from build123d import *

# Parameters (mm, degrees)
SKETCH1_R           = 1.725
SKETCH1_R_2         = 3
BOSS_EXTRUDE3_DEPTH = 6
CUT_EXTRUDE1_DEPTH  = 4
FILLET1_R           = 4


with BuildPart() as part:
    # Sketch1 → Boss-Extrude3 (new body)
    with BuildSketch(Plane.XY):
        with BuildLine():
            ThreePointArc((22.418161887, -16.775756842), (28, 0), (22.418161887, 16.775756842))
            ThreePointArc((22.418161887, 16.775756842), (22.627416998, 22.627416998), (16.775756842, 22.418161887))
            ThreePointArc((16.775756842, 22.418161887), (0, 28), (-16.775756842, 22.418161887))
            ThreePointArc((-16.775756842, 22.418161887), (-22.627416998, 22.627416998), (-22.418161887, 16.775756842))
            ThreePointArc((-22.418161887, 16.775756842), (-28, 0), (-22.418161887, -16.775756842))
            ThreePointArc((-22.418161887, -16.775756842), (-22.627416998, -22.627416998), (-16.775756842, -22.418161887))
            ThreePointArc((-16.775756842, -22.418161887), (0, -28), (16.775756842, -22.418161887))
            ThreePointArc((16.775756842, -22.418161887), (22.627416998, -22.627416998), (22.418161887, -16.775756842))
        make_face()
        with Locations((-19.798989873, 19.798989873)):
            Circle(SKETCH1_R, mode=Mode.SUBTRACT)
        with Locations((19.798989873, 19.798989873)):
            Circle(SKETCH1_R, mode=Mode.SUBTRACT)
        with Locations((-19.798989873, -19.798989873)):
            Circle(SKETCH1_R, mode=Mode.SUBTRACT)
        with Locations((19.798989873, -19.798989873)):
            Circle(SKETCH1_R, mode=Mode.SUBTRACT)
        Circle(SKETCH1_R_2, mode=Mode.SUBTRACT)
        with Locations((0, 7.5)):
            Circle(SKETCH1_R, mode=Mode.SUBTRACT)
        with Locations((-7.5, 0)):
            Circle(SKETCH1_R, mode=Mode.SUBTRACT)
        with Locations((0, -7.5)):
            Circle(SKETCH1_R, mode=Mode.SUBTRACT)
        with Locations((7.5, 0)):
            Circle(SKETCH1_R, mode=Mode.SUBTRACT)
    extrude(amount=BOSS_EXTRUDE3_DEPTH)

    # Sketch2 → Cut-Extrude1 (cut)
    with BuildSketch(Plane.XY.offset(6)):
        Polygon((3.290896534, 7.5), (1.645448267, 10.35), (-1.645448267, 10.35), (-3.290896534, 7.5), (-1.645448267, 4.65), (1.645448267, 4.65), align=None)
        Polygon((-4.65, 1.645448267), (-7.5, 3.290896534), (-10.35, 1.645448267), (-10.35, -1.645448267), (-7.5, -3.290896534), (-4.65, -1.645448267), align=None)
        Polygon((10.35, -1.645448267), (10.35, 1.645448267), (7.5, 3.290896534), (4.65, 1.645448267), (4.65, -1.645448267), (7.5, -3.290896534), align=None)
        Polygon((3.290896534, -7.5), (1.645448267, -4.65), (-1.645448267, -4.65), (-3.290896534, -7.5), (-1.645448267, -10.35), (1.645448267, -10.35), align=None)
    extrude(amount=-CUT_EXTRUDE1_DEPTH, mode=Mode.SUBTRACT)

    # Fillet1
    fillet1_edges = [part.edges().sort_by_distance(p)[0] for p in [
        (22.418161887, 16.775756842, 3),
        (22.418161887, -16.775756842, 3),
        (16.775756842, -22.418161887, 3),
        (-16.775756842, -22.418161887, 3),
        (-22.418161887, -16.775756842, 3),
        (-22.418161887, 16.775756842, 3),
        (-16.775756842, 22.418161887, 3),
        (16.775756842, 22.418161887, 3),
    ]]
    fillet(fillet1_edges, radius=FILLET1_R)


solid = part.part
Can you work these out from the model? Positions are in its coordinate system, mm. A direction names the side the tool comes from. Coordinates: 2 decimals unless noted, no trailing zeros. Write each loop counter-clockwise with the first axis right and the second up, starting at its lowest first coordinate (ties: lowest second). Pieces come first, ordered by that corner, then holes. Notation, with made-up numbers: (38.5, 78.5) -> (49.5, 78.5) arc R31 ccw to (49.5, 102.5) -> close; hole circle Ø6 at (-22.5, -8). An arc over 180 degrees is marked (long way). Write each question's results on one line, items separated by ' | '. Start each with the question number.
Item 1: Thinking about a two-plate mould opening in Y: for faces 3 (the flat face through (6, -6, 0)), 4 (the flat face through (-8.94, -2.46, 4.03)), 5 (the cylindrical face through (0, 28, 3)), 6 (the flat face through (-6.06, 2.46, 4.03)), which applies, released by +Y, released by -Y, zero draft, split by the parting line, or undercut?
Item 2: If we section it at B-B, the plane x = 6.5: Write out the boundary of the cut face in (y, z), and give its area (3 significant figures).
Item 3: If we section it at C-C, the plane y = 1: Write out the boundary of the cut face in (x, z), and give its area (3 significant figures).
Item 4: Please list where these lines run through material, in increasing order: probe 1 along Y at (x, z) = (0, 0.8) (3 decimals); probe 2 along Y at (x, z) = (0, 2.6); probe 3 along X at (y, z) = (1, 5.5).
Item 5: If we section it at A-A, the plane x = 0: Write out the boundary of the cut face in (y, z) (3 decimals).
Item 6: I'm going to push flat-ended pins straight in: P1, Ø3.5, axis at x = -1, z = 4.5, coming from the -Y side; P2, Ø2.5, axis at x = -0.5, z = 4, coming from the +Y side; P3, Ø3, axis at y = 20.5, z = 4.5, coming from the +X side. Where does each tip first touch, or does it pass through?
Item 7: On a 3-axis mill with a long thin cutter (end or side, diameter ignored), from which of +Z, -Z, +X, -X, +Y, -Y can I reach the whole of each face in a straight line? I mean faces 1 (the cylindrical face through (-19, 18.27, 2.96)), 2 (the flat face through (0, -10.35, 4)). Say none if no direction works.
Item 8: If we section it at D-D, the plane z = 4.25: Count the separate pieces of the cut face and the enclosed holes in it, and give its area (3 significant figures).
Answer block:
1) face 3: zero draft | face 4: undercut | face 5: released by +Y | face 6: undercut
2) outline: (-27.24, 0) -> (-1.41, 0) -> (-1.41, 2) -> (-2.71, 2) -> (-2.71, 6) -> (-27.24, 6) -> close; (1.41, 0) -> (27.24, 0) -> (27.24, 6) -> (2.71, 6) -> (2.71, 2) -> (1.41, 2) -> close | area: 299 mm²
3) outline: (-27.98, 0) -> (-8.91, 0) -> (-8.91, 2) -> (-10.35, 2) -> (-10.35, 6) -> (-27.98, 6) -> close; (-6.09, 0) -> (-2.83, 0) -> (-2.83, 6) -> (-4.65, 6) -> (-4.65, 2) -> (-6.09, 2) -> close; (2.83, 0) -> (6.09, 0) -> (6.09, 2) -> (4.65, 2) -> (4.65, 6) -> (2.83, 6) -> close; (8.91, 0) -> (27.98, 0) -> (27.98, 6) -> (10.35, 6) -> (10.35, 2) -> (8.91, 2) -> close | area: 245 mm²
4) probe 1: -28 to -9.225, -5.775 to -3, 3 to 5.775, 9.225 to 28 | probe 2: -28 to -10.35, -4.65 to -3, 3 to 4.65, 10.35 to 28 | probe 3: -27.98 to -10.35, -4.65 to -2.83, 2.83 to 4.65, 10.35 to 27.98
5) outline: (-28, 0) -> (-9.225, 0) -> (-9.225, 2) -> (-10.35, 2) -> (-10.35, 6) -> (-28, 6) -> close; (-5.775, 0) -> (-3, 0) -> (-3, 6) -> (-4.65, 6) -> (-4.65, 2) -> (-5.775, 2) -> close; (3, 0) -> (5.775, 0) -> (5.775, 2) -> (4.65, 2) -> (4.65, 6) -> (3, 6) -> close; (9.225, 0) -> (28, 0) -> (28, 6) -> (10.35, 6) -> (10.35, 2) -> (9.225, 2) -> close
6) P1: y = -28 | P2: y = 28 | P3: x = 23.8
7) face 1: +Z, -Z | face 2: +Z
8) separate pieces: 1 | enclosed holes: 9 | area: 2,400 mm²
